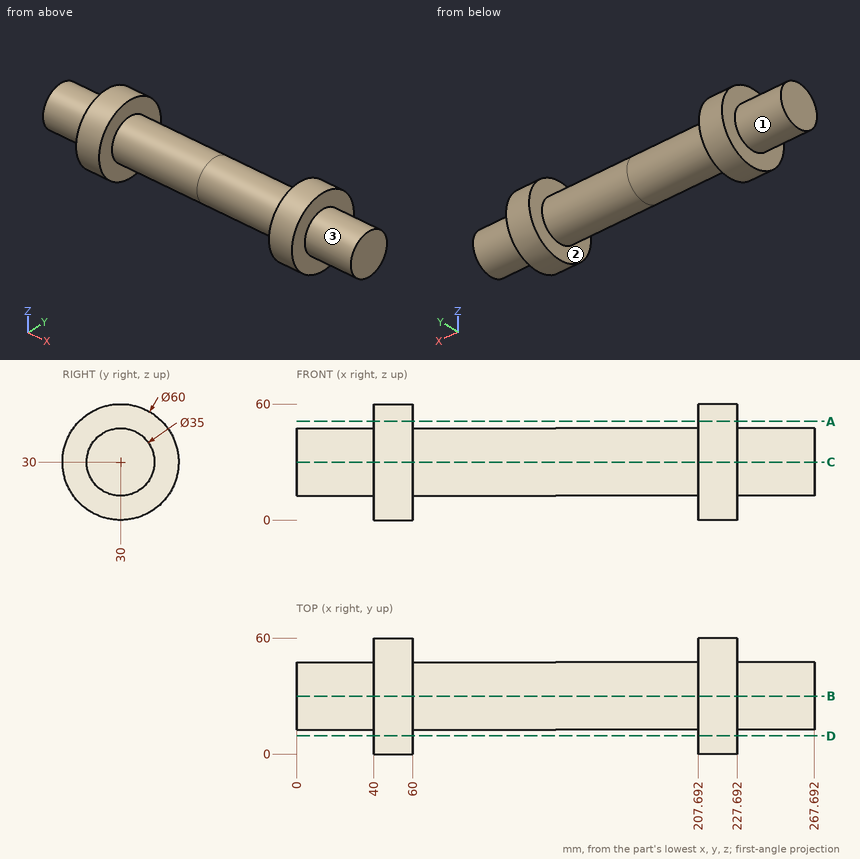
Geometry check sheet. Reference: drawing and pictorial views, mm from the part's lowest x, y, z. A direction names the side the tool comes from. Coordinates: 2 decimals unless noted, no trailing zeros. Order: outer loops, then holes, each group sorted by start corner. A loop starts at its lowest first (then second) coordinate and runs counter-clockwise, first axis right, second up.
Item 1: Tool access check on the marked faces 1, 2 and 3. Record the directions out of +Z, -Z, +X, -X, +Y, -Y that give a thin tool (end or side, any length) a straight path to the whole face; none if there is none.
Item 2: Scan lines: line 1 along X through (y, z) = (17, 50); line 2 along Y through (x, z) = (133, 30.5); line 3 along Z through (x, y) = (256, 29). Record each from-to range of solid material in increasing order.
Item 3: Depth check by flat-ended pin: pin 1 (12 mm diameter, centred on x = 234.5, z = 32.5, fed in from -Y); pin 2 (1.5 mm diameter, centred on x = 212.5, y = 17.5, fed in from -Z); pin 3 (8 mm diameter, centred on x = 31.5, y = 30.5, fed in from -Z). Enter the tip coordinate at first touch or a pass-through.
Item 4: Section check B-B (y = 30). Enter the section's corners in (x, z).
Item 5: Section check A-A (z = 51). Enter the section's corners in (x, y), plus the area to 3 significant figures.
Item 6: Section check D-D (y = 9.5). Enter the section's corners in (x, z).
Check sheet entries:
1. face 1: -X
1. face 2: none
1. face 3: +X
2. line 1: x = 40 to 60, 207.69 to 227.69
2. line 2: y = 12.51 to 47.49
2. line 3: z = 12.53 to 47.47
3. pin 1: stops at y = 12.5
3. pin 2: stops at z = 2.4
3. pin 3: stops at z = 12.5
4. outline: (0, 12.5) - (40, 12.5) - (40, 0) - (60, 0) - (60, 12.5) - (207.69, 12.5) - (207.69, 0) - (227.69, 0) - (227.69, 12.5) - (267.69, 12.5) - (267.69, 47.5) - (227.69, 47.5) - (227.69, 60) - (207.69, 60) - (207.69, 47.5) - (60, 47.5) - (60, 60) - (40, 60) - (40, 47.5) - (0, 47.5) - close
5. outline: (40, 8.58) - (60, 8.58) - (60, 51.42) - (40, 51.42) - close; (207.69, 8.58) - (227.69, 8.58) - (227.69, 51.42) - (207.69, 51.42) - close
5. area: 1,710 mm2
6. outline: (40, 8.1) - (60, 8.1) - (60, 51.9) - (40, 51.9) - close; (207.69, 8.1) - (227.69, 8.1) - (227.69, 51.9) - (207.69, 51.9) - close
